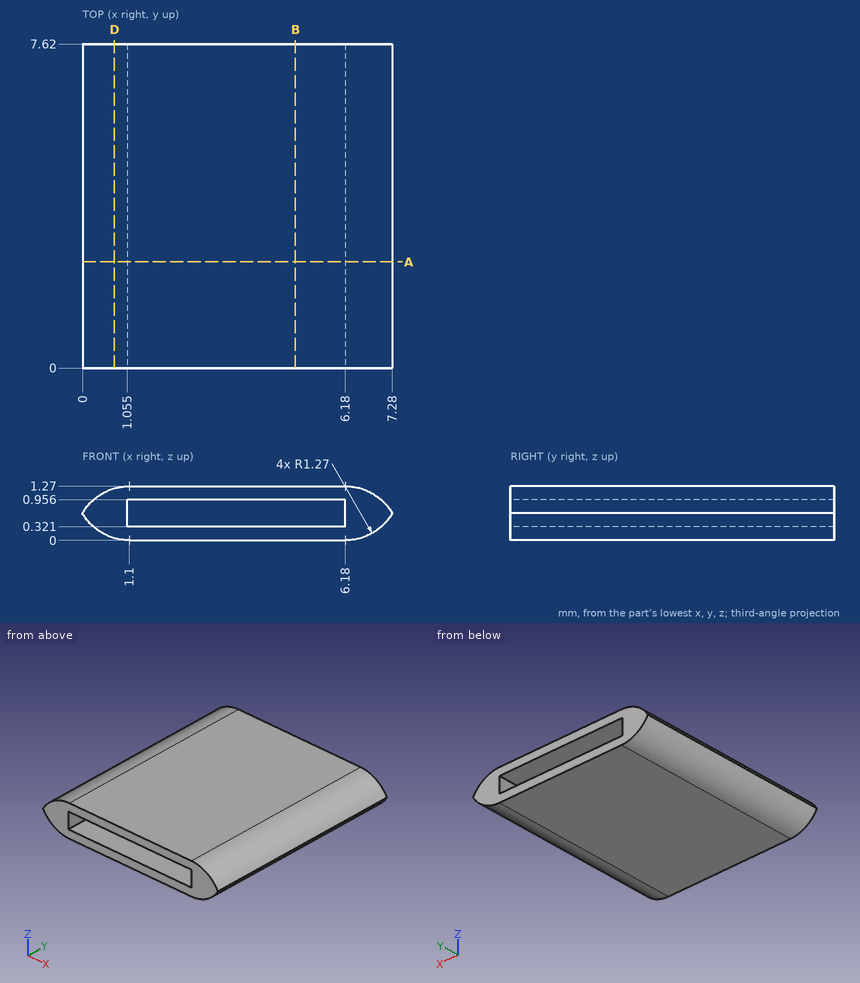
Check sheet for the drawn part. Datum: minimum x, y, z corner. Units: mm. Give positions to 0.01 mm unless a question says otherwise; leave off trailing zeros. Order: outer loops, then holes, each group sorted by start corner. A loop starts at its lowest first (then second) coordinate and runs counter-clockwise, first axis right, second up. Notation, with made-up numbers: (11.5, 8) - (56.5, 8) arc R26 cw to (56.5, 43) - close; hole circle Ø8 at (-3, 47.5). An arc over 180 degrees is marked (long way). Answer as a JSON object with one key per item and string values.
(1) Cross-section at B-B (x = 5). Record the cut outline in (y, z).
Report:
{"outline": "(0, 0) - (7.62, 0) - (7.62, 0.32) - (0, 0.32) - close; (0, 0.96) - (7.62, 0.96) - (7.62, 1.27) - (0, 1.27) - close"}
(2) Cross-section at D-D (x = 0.75). Record the cut outline in (y, z).
Report:
{"outline": "(0, 0.05) - (7.62, 0.05) - (7.62, 1.22) - (0, 1.22) - close"}
(3) Material ranges on line 1 (Z direction, x = 5, y = 5); line 2 (X direction, y = 3.25, z = 0.8) (1 decimal); line 3 (X direction, y = 2, z = 0.7) (1 decimal), recorded low to high.
Report:
{"line 1": "0 to 0.32, 0.96 to 1.27", "line 2": "0.1 to 1.1, 6.2 to 7.2", "line 3": "0 to 1.1, 6.2 to 7.2"}
(4) Cross-section at A-A (y = 2.5). Record the cut outline in (x, z) (1 decimal).
Report:
{"outline": "(0, 0.6) arc R1.3 ccw to (1.1, 0) - (6.2, 0) arc R1.3 ccw to (7.3, 0.6) arc R1.3 ccw to (6.2, 1.3) - (1.1, 1.3) arc R1.3 ccw to start; hole (1.1, 0.3) - (6.2, 0.3) - (6.2, 1) - (1.1, 1) - close"}
